```python
from build123d import *

# Parameters (mm, degrees)
F1_DEPTH      = 28.75
F3_DEPTH      = 105.001
F3_DEPTH_BACK = 105.001
F4_T1_DEPTH   = 100
F5_R          = 5
F7_D          = 30


# Not quite as in the source:
# - a fillet or chamfer that OpenCascade refuses, or shapes differently, is made with other operations: its cross-section is extruded or revolved along the edge and cut away or added


with BuildPart() as f1:
    # F0 (on Front) → F1 (new body, symmetric)
    with BuildSketch(Plane.XZ):
        with BuildLine():
            Line((-105, 30), (-105, 0))
            Line((-105, 0), (105, 0))
            Line((105, 0), (105, 30))
            Line((105, 30), (50, 30))
            Line((50, 30), (50, 172.5))
            Line((50, 172.5), (58, 172.5))
            Line((58, 172.5), (58, 217.5))
            Line((58, 217.5), (50, 217.5))
            Line((50, 217.5), (50, 315))
            Line((50, 315), (-50, 315))
            Line((-50, 315), (-50, 235))
            Line((-50, 235), (10, 235))
            ThreePointArc((10, 235), (50, 195), (10, 155))
            Line((10, 155), (-50, 155))
            Line((-50, 155), (-50, 30))
            Line((-50, 30), (-105, 30))
        make_face()
    extrude(amount=F1_DEPTH, both=True)

    # F2 (on Right) → F3 (cut, two sides)
    with BuildSketch(Plane.YZ) as f3_sk:
        with BuildLine():
            Line((-129.573866725, 348.6788272858), (-129.573866725, 30))
            Line((-129.573866725, 30), (-20, 30))
            Line((-20, 30), (-20, 70))
            Line((-20, 70), (-28.75, 70))
            Line((-28.75, 70), (-28.75, 306.3482712035))
            ThreePointArc((-28.75, 306.3482712035), (0, 310), (28.75, 306.3482712035))
            Line((28.75, 306.3482712035), (28.75, 70))
            Line((28.75, 70), (20, 70))
            Line((20, 70), (20, 30))
            Line((20, 30), (130.780075267, 30))
            Line((130.780075267, 30), (130.780075267, 348.6788272858))
            Line((130.780075267, 348.6788272858), (-129.573866725, 348.6788272858))
        make_face()
    extrude(amount=-F3_DEPTH, mode=Mode.SUBTRACT)
    extrude(f3_sk.sketch, amount=F3_DEPTH_BACK, mode=Mode.SUBTRACT)

    # F4: fillet of radius 20 on 2 edges, made by hand

    # F4_s2 → F4_t1 (join)
    with BuildSketch(Plane.YZ.offset(-50)):
        with BuildLine():
            ThreePointArc((-20, 46.5359456942), (-22.3223304703, 37.1818022272), (-28.75, 30))
            Line((-28.75, 30), (-20, 30))
            Line((-20, 30), (-20, 46.5359456942))
        make_face()
        with BuildLine():
            ThreePointArc((20, 46.5359456942), (22.3223304703, 37.1818022272), (28.75, 30))
            Line((28.75, 30), (20, 30))
            Line((20, 30), (20, 46.5359456942))
        make_face()
    extrude(amount=F4_T1_DEPTH)

    # F5
    f5_edges = [f1.edges().sort_by_distance(p)[0] for p in [
        (0, 20, 70),
        (0, -20, 70),
    ]]
    fillet(f5_edges, radius=F5_R)

    # F7 (through all)
    with Locations(Plane(origin=(-50, 0, 0), x_dir=(0, -1, 0), z_dir=(-1, 0, 0))):
        with Locations((0, 270), (0, 120)):
            Hole(F7_D / 2)


solid = f1.part
```
Could you check a few things on this model? Use its own coordinates, in mm. A direction names the side the tool comes from. Give positions to 0.01 mm unless a question says otherwise; leave off trailing zeros. Loops run counter-clockwise (first coordinate to the right, second up) from the corner with the lowest first, then second, coordinate; pieces in that order, holes last. Notation, with made-up numbers: (-2, 1) - (30, 1) arc R31 ccw to (30, 37) - close; hole circle Ø6 at (9.5, 74). An arc over 180 degrees is marked (long way). Answer in a Markdown table with one row per item. Add a question column.
Q1. If we section it at B-B (z = 270): List the corners of the cut face in (x, y) for me.
Q2. If we section it at C-C (z = 195): List the corners of the cut face in (x, y) for me, plus the area to 3 significant figures.
Q3. If we section it at D-D (x = 68.5): List the corners of the cut face in (y, z) for me.
Q4. For pin 1 (9 mm diameter, centred on x = 10, z = 60, fed in from -Y); pin 2 (4 mm diameter, centred on x = 41, y = 14.5, fed in from +Z); pin 3 (12 mm diameter, centred on y = 10, z = 36.5, fed in from +X), each with a flat end and sliding along its axis, tell me the tip position at first contact or that it passes through.
Q5. Which directions (+Z, -Z, +X, -X, +Y, -Y) give clear straight access to the entire face, cutting with the end or side of a thin tool? Please do faces 1 (the face through (58, 0, 195)), 2 (the face through (50, 0, 102)), 3 (the face through (-20, 0, 155)), 4 (the face through (-77, 0, 30)).
Q6. Please list where these lines run through material, in increasing order: L1, parallel to Z at x = -27, y = 0; L2, parallel to Z at x = 18, y = 0; L3, parallel to X at y = 7, z = 139.5. Write a range as from..to.
Q7. We'd pull the mould along Z, two halves only. Please class faces 5 (the face through (-1, 0, 310)), 6 (the face through (0.7, -1.953, 284.872)), 7 (the face through (50, 0, 253)): +Z half, -Z half, draft (parallel to the pull), parting line (faces both ways), or undercut.
Q8. If we section it at A-A (y = 0): List the corners of the cut face in (x, z) for me.
The answers:
| question | item | result |
|---|---|---|
| 1 | outline | (-50, -28.75) - (50, -28.75) - (50, -15) - (-50, -15) - close; (-50, 15) - (50, 15) - (50, 28.75) - (-50, 28.75) - close |
| 2 | outline | (50, -28.75) - (58, -28.75) - (58, 28.75) - (50, 28.75) - close |
| 2 | area | 460 mm^2 |
| 3 | outline | (-28.75, 0) - (28.75, 0) - (28.75, 30) - (-28.75, 30) - close |
| 4 | pin 1 | stops at y = -20 |
| 4 | pin 2 | stops at z = 309.32 |
| 4 | pin 3 | stops at x = 50 |
| 5 | face 1 | +Z, +X, +Y, -Y |
| 5 | face 2 | +X, +Y, -Y |
| 5 | face 3 | -X, +Y, -Y |
| 5 | face 4 | +Z, -X, +Y, -Y |
| 6 | L1 | z = 0..105, 135..155, 235..255, 285..310 |
| 6 | L2 | z = 0..105, 135..155.81, 234.19..255, 285..310 |
| 6 | L3 | x = -50..50 |
| 7 | face 5 | +Z half |
| 7 | face 6 | undercut |
| 7 | face 7 | draft |
| 8 | outline | (-105, 0) - (105, 0) - (105, 30) - (50, 30) - (50, 105) - (-50, 105) - (-50, 30) - (-105, 30) - close; (-50, 135) - (50, 135) - (50, 172.5) - (58, 172.5) - (58, 217.5) - (50, 217.5) - (50, 255) - (-50, 255) - (-50, 235) - (10, 235) arc R40 cw to (10, 155) - (-50, 155) - close; (-50, 285) - (50, 285) - (50, 310) - (-50, 310) - close |
